from build123d import *

# Parameters (mm, degrees)
SKETCH1_R           = 2.38125
EXTRUDE1_DEPTH      = 7.7390625
FILLET1_R           = 1.016
EXTRUDE2_DEPTH      = 9.440011345
EXTRUDE2_DEPTH_BACK = 9.440011345
SKETCH4_W           = 0.5953125
SKETCH4_H           = 1.190625


with BuildPart() as part:
    # Sketch1 → Extrude1 (new, symmetric)
    with BuildSketch(Plane.XY):
        Circle(SKETCH1_R)
    extrude(amount=EXTRUDE1_DEPTH, both=True)

    # Fillet1
    fillet1_edges = [part.edges().sort_by_distance(p)[0] for p in [
        (-2.38125, 0, -7.7390625),
        (-2.38125, 0, 7.7390625),
    ]]
    fillet(fillet1_edges, radius=FILLET1_R)

    # Sketch3 → Extrude2 (cut, two sides: drawn at the far end of the back side and taken through both)
    with BuildSketch(Plane.XY.offset(-EXTRUDE2_DEPTH_BACK)):
        with BuildLine():
            Line((-0.9921875, 2.16469756), (-0.9921875, 1.1191875))
            ThreePointArc((-0.9921875, 1.1191875), (-1.029384939, 1.029384939), (-1.1191875, 0.9921875))
            Line((-1.1191875, 0.9921875), (-2.16469756, 0.9921875))
            ThreePointArc((-2.16469756, 0.9921875), (-1.683798023, 1.683798023), (-0.9921875, 2.16469756))
        make_face()
        with BuildLine():
            Line((-2.16469756, -0.9921875), (-1.1191875, -0.9921875))
            ThreePointArc((-1.1191875, -0.9921875), (-1.029384939, -1.029384939), (-0.9921875, -1.1191875))
            Line((-0.9921875, -1.1191875), (-0.9921875, -2.16469756))
            ThreePointArc((-0.9921875, -2.16469756), (-1.683798023, -1.683798023), (-2.16469756, -0.9921875))
        make_face()
        with BuildLine():
            Line((0.9921875, 2.16469756), (0.9921875, 1.1191875))
            ThreePointArc((0.9921875, 1.1191875), (1.029384939, 1.029384939), (1.1191875, 0.9921875))
            Line((1.1191875, 0.9921875), (2.16469756, 0.9921875))
            ThreePointArc((2.16469756, 0.9921875), (1.683798023, 1.683798023), (0.9921875, 2.16469756))
        make_face()
        with BuildLine():
            Line((0.9921875, -1.1191875), (0.9921875, -2.16469756))
            ThreePointArc((0.9921875, -2.16469756), (1.683798023, -1.683798023), (2.16469756, -0.9921875))
            Line((2.16469756, -0.9921875), (1.1191875, -0.9921875))
            ThreePointArc((1.1191875, -0.9921875), (1.029384939, -1.029384939), (0.9921875, -1.1191875))
        make_face()
    extrude(amount=EXTRUDE2_DEPTH + EXTRUDE2_DEPTH_BACK, mode=Mode.SUBTRACT)

    # Sketch4 → Cut-Revolve1 (revolve, cut)
    with BuildSketch(Plane(origin=(0, 0, 0), x_dir=(1, 0, 0), z_dir=(0, 1, 0))):
        with Locations((-2.08359375, 4.9609375)):
            Rectangle(SKETCH4_W, SKETCH4_H)
        with Locations((-2.08359375, -4.9609375)):
            Rectangle(SKETCH4_W, SKETCH4_H)
    revolve(axis=Axis((0, 0, -7.7390625), (0, 0, 1)), mode=Mode.SUBTRACT)


solid = part.part
Work out the finished part from the listing and answer in its coordinate system (mm). A direction names the side the tool comes from. Coordinates: 2 decimals unless noted, no trailing zeros. Write each loop counter-clockwise with the first axis right and the second up, starting at its lowest first coordinate (ties: lowest second). Pieces come first, ordered by that corner, then holes.
1. The part is cut by section B-B, the plane y = 1.95. State how many separate pieces and enclosed holes the cut face has, and give its area (3 significant figures).
Results list:
separate pieces: 3
enclosed holes: 0
area: 25.0 mm2
2. Flat-ended cylindrical pins translate along their axes: pin 1 (0.8 mm diameter, centred on y = 2, z = -2.5, fed in from -X); pin 2 (0.5 mm diameter, centred on y = -1.5, z = 2.5, fed in from +X); pin 3 (0.7 mm diameter, centred on x = 2, y = 0.5, fed in from +Z). Find the tip coordinate at first contact, or state that the pin passes through.
Results list:
pin 1: stops at x = -0.99
pin 2: stops at x = 0.99
pin 3: stops at z = 7.68
3. Consider line 1 along Z through (x, y) = (0.9, -1.8); line 2 along Z through (x, y) = (1.8, -0.75); line 3 along X through (y, z) = (1.35, -5.5). Determine where each line is inside the solid, lowest interval first.
Results list:
line 1: z = -7.51 to -5.56, -4.37 to 4.37, 5.56 to 7.51
line 2: z = -7.55 to -5.56, -4.37 to 4.37, 5.56 to 7.55
line 3: x = -0.99 to 0.99
4. For a pull along Z with two mould halves and no side action, classify faces 1 (the flat face through (0, 0, 7.739)), 2 (the cylindrical face through (-0.01, -2.38, 6.15)), 3 (the cylindrical face through (-1.786, 0.015, 4.953)) as +Z half, -Z half, draft (parallel to the pull), parting line (faces both ways), or undercut.
Results list:
face 1: +Z half
face 2: draft
face 3: undercut
5. The part is cut by section A-A, the plane z = 4. Write down the section's boundary in (x, y).
Results list:
outline: (-2.16, -0.99) - (-1.12, -0.99) arc R0.13 cw to (-0.99, -1.12) - (-0.99, -2.16) arc R2.38 ccw to (0.99, -2.16) - (0.99, -1.12) arc R0.13 cw to (1.12, -0.99) - (2.16, -0.99) arc R2.38 ccw to (2.16, 0.99) - (1.12, 0.99) arc R0.13 cw to (0.99, 1.12) - (0.99, 2.16) arc R2.38 ccw to (-0.99, 2.16) - (-0.99, 1.12) arc R0.13 cw to (-1.12, 0.99) - (-2.16, 0.99) arc R2.38 ccw to start
6. For faces 4 (the cylindrical face through (-0.015, -1.786, 4.953)), 5 (the flat face through (-2, 0.992, 0)), 6 (the cylindrical face through (0.015, 1.786, -4.969)), 7 (the flat face through (0.992, -2, 0)), 8 (the flat face through (0.992, 2, 0)), determine the directions among +Z, -Z, +X, -X, +Y, -Y from which every point of the face is accessible in a straight line to the end or side of a thin tool.
Results list:
face 4: -Y
face 5: +Z, -Z, -X, +Y
face 6: +Y
face 7: +Z, -Z, +X, -Y
face 8: +Z, -Z, +X, +Y
